Verification items for the finished model (mm, model axes). A direction names the side the tool comes from. Coordinates: 2 decimals unless noted, no trailing zeros. Order: outer loops, then holes, each group sorted by start corner. A loop starts at its lowest first (then second) coordinate and runs counter-clockwise, first axis right, second up. Notation, with made-up numbers: (12.25, 77.5) -> (40.25, 77.5) arc R20 ccw to (40.25, 105.5) -> close; hole circle Ø1 at (21.25, 59). An arc over 180 degrees is marked (long way). Write item = value, one per line. Start each with the question number.
1. Cross-section at B-B on x = 2.6. Record the cut outline in (y, z).
2. Go/stop test with flat-tipped pins: P1, Ø1, axis at y = -5.5, z = 0, coming from the -X side; P2, Ø0.5, axis at y = -4.5, z = -5, coming from the +X side; P3, Ø3.5, axis at y = 6.5, z = -3, coming from the +X side. Record where each tip stops, or that it passes through.
3. Cross-section at A-A on y = -1.75. Record the cut outline in (x, z), plus the area to 3 significant figures.
4. Cross-section at C-C on z = -3.25. Record the cut outline in (x, y).
5. Thickness scan on line 1 along Y through (x, z) = (-0.4, -3.25); line 2 along X through (y, z) = (7, -4.75); line 3 along Y through (x, z) = (-0.65, 2). Record the ranges inside material, lowest first. Write a range as from..to.
6. Release check for a two-part mould opening along Y. For faces 5 (the cylindrical face through (0.04, -1.73, 2.15)), 6 (the flat face through (-0.2, -5, 5)), 7 (the flat face through (0.028, 3.933, 1.174)) record: +Y half, -Y half, draft (parallel to the pull), parting line (faces both ways), or undercut.
7. Set-up check for faces 1 (the flat face through (0, 0, 6.4)), 2 (the flat face through (0.2, -5, 0)), 3 (the flat face through (-0.2, -5, -5)), 4 (the cylindrical face through (0.03, 7.53, -6.25)): record each of +Z, -Z, +X, -X, +Y, -Y from which the full face is reachable in a straight line by a thin tool's end or side.
8. Cross-section at D-D on x = -1. Record the cut outline in (y, z), plus the area to 3 significant figures.
from build123d import *

# Parameters (mm, degrees)
SKETCH1_W           = 12.8
SKETCH1_H           = 6.5
SKETCH1_R           = 1
BOSS_EXTRUDE1_DEPTH = 3
SKETCH3_W           = 0.9
SKETCH3_H           = 4
BOSS_EXTRUDE2_DEPTH = 0.2
BOSS_EXTRUDE3_DEPTH = 2
FILLET1_R           = 0.2
BOSS_EXTRUDE5_DEPTH = 0.5


with BuildPart() as part:
    # Sketch1 → Boss-Extrude1 (new body, symmetric)
    with BuildSketch(Plane(origin=(0, 0, 0), x_dir=(0, 0, -1), z_dir=(1, 0, 0))):
        Rectangle(SKETCH1_W, SKETCH1_H)
        with Locations((3.25, -1.75)):
            Circle(SKETCH1_R, mode=Mode.SUBTRACT)
        with BuildLine():
            Line((-3.708257569, -0.75), (-2.791742431, -0.75))
            ThreePointArc((-2.791742431, -0.75), (-2.15, -1.75), (-2.791742431, -2.75))
            Line((-2.791742431, -2.75), (-3.708257569, -2.75))
            ThreePointArc((-3.708257569, -2.75), (-4.35, -1.75), (-3.708257569, -0.75))
        make_face(mode=Mode.SUBTRACT)
    extrude(amount=BOSS_EXTRUDE1_DEPTH, both=True)

    # Sketch3 → Boss-Extrude2 (add, symmetric)
    with BuildSketch(Plane(origin=(0, 0, 0), x_dir=(0, 0, -1), z_dir=(1, 0, 0))):
        with Locations((-5.08, -5.25)):
            Rectangle(SKETCH3_W, SKETCH3_H)
        with Locations((0, -5.25)):
            Rectangle(SKETCH3_W, SKETCH3_H)
        with Locations((5.08, -5.25)):
            Rectangle(SKETCH3_W, SKETCH3_H)
    extrude(amount=BOSS_EXTRUDE2_DEPTH, both=True)

    # Sketch4 → Boss-Extrude3 (add, symmetric)
    with BuildSketch(Plane(origin=(0, 0, 0), x_dir=(0, 0, -1), z_dir=(1, 0, 0))):
        with BuildLine():
            Line((-5.9, 3.25), (3.877784075, 4.663655529))
            ThreePointArc((3.877784075, 4.663655529), (6.163655529, 7.722215925), (9.222215925, 5.436344471))
            Line((9.222215925, 5.436344471), (9.024274005, 5.407726362))
            ThreePointArc((9.024274005, 5.407726362), (6.093510034, 7.507970079), (4.11227449, 4.495478279))
            Line((4.11227449, 4.495478279), (-4.502283608, 3.25))
            Line((-4.502283608, 3.25), (-5.9, 3.25))
        make_face()
    extrude(amount=BOSS_EXTRUDE3_DEPTH, both=True)

    # Fillet1
    fillet1_edges = [part.edges().sort_by_distance(p)[0] for p in [
        (0, 4.495478279, -4.11227449),
        (0, 4.663655529, -3.877784075),
    ]]
    fillet(fillet1_edges, radius=FILLET1_R)

    # Sketch5 → Boss-Extrude5 (add, symmetric)
    with BuildSketch(Plane(origin=(0, 0, 0), x_dir=(0, 0, -1), z_dir=(1, 0, 0))):
        with BuildLine():
            Line((-2.48, 3.25), (-1.82, 3.25))
            ThreePointArc((-1.82, 3.25), (-2.15, 3.58), (-2.48, 3.25))
        make_face()
    extrude(amount=BOSS_EXTRUDE5_DEPTH, both=True)


solid = part.part
Worked out:
q1.outline = (-3.25, -6.4) -> (3.25, -6.4) -> (3.25, 6.4) -> (-3.25, 6.4) -> close; hole circle Ø2 at (-1.75, -3.25); hole (-2.75, 2.79) arc R1.1 ccw to (-0.75, 2.79) -> (-0.75, 3.71) arc R1.1 ccw to (-2.75, 3.71) -> close
q2.P1 = -0.2
q2.P2 = 0.2
q2.P3 = 2
q3.outline = (-3, -6.4) -> (3, -6.4) -> (3, -4.25) -> (-3, -4.25) -> close; (-3, -2.25) -> (3, -2.25) -> (3, 2.15) -> (-3, 2.15) -> close; (-3, 4.35) -> (3, 4.35) -> (3, 6.4) -> (-3, 6.4) -> close
q3.area = 51.6 mm²
q4.outline = (-3, -3.25) -> (3, -3.25) -> (3, -2.75) -> (-3, -2.75) -> close; (-3, -0.75) -> (3, -0.75) -> (3, 3.25) -> (-3, 3.25) -> close; (-2, 4.37) -> (2, 4.37) -> (2, 4.57) -> (-2, 4.57) -> close
q5.line_1 = -3.25..-2.75, -0.75..3.25, 4.37..4.57
q5.line_2 = -2..2
q5.line_3 = -3.25..3.25, 3.61..3.81
q6.face_5 = undercut
q6.face_6 = draft
q6.face_7 = +Y half
q7.face_1 = +Z, +X, -X, +Y, -Y
q7.face_2 = +Z, -Z, +X, -Y
q7.face_3 = +Z, -Z, -X, -Y
q7.face_4 = +X, -X
q8.outline = (-3.25, -6.4) -> (3.25, -6.4) -> (3.25, 4.5) -> (4.47, -3.91) arc R0.2 ccw to (4.69, -4.08) arc R2.5 cw to (5.41, -9.02) -> (5.44, -9.22) arc R2.7 ccw to (4.85, -3.86) arc R0.2 cw to (4.64, -3.69) -> (3.25, 5.9) -> (3.25, 6.4) -> (-3.25, 6.4) -> close; hole circle Ø2 at (-1.75, -3.25); hole (-2.75, 2.79) arc R1.1 ccw to (-0.75, 2.79) -> (-0.75, 3.71) arc R1.1 ccw to (-2.75, 3.71) -> close
q8.area = 79.9 mm²
